The drawing under review shows one solid part. Ordinate dimensions are in mm from its lowest x, y, z. A direction names the side the tool comes from. Round coordinates to 2 decimals unless told otherwise and drop trailing zeros. Write each loop counter-clockwise with the first axis right and the second up, starting at its lowest first coordinate (ties: lowest second). Pieces come first, ordered by that corner, then holes. Notation, with made-up numbers: (-22.75, -29) -> (12.25, -29) arc R13 ccw to (12.25, -9) -> close; hole circle Ø4 at (83, 34.25). An arc over 180 degrees is marked (long way). Answer in a Markdown table with one row per item.
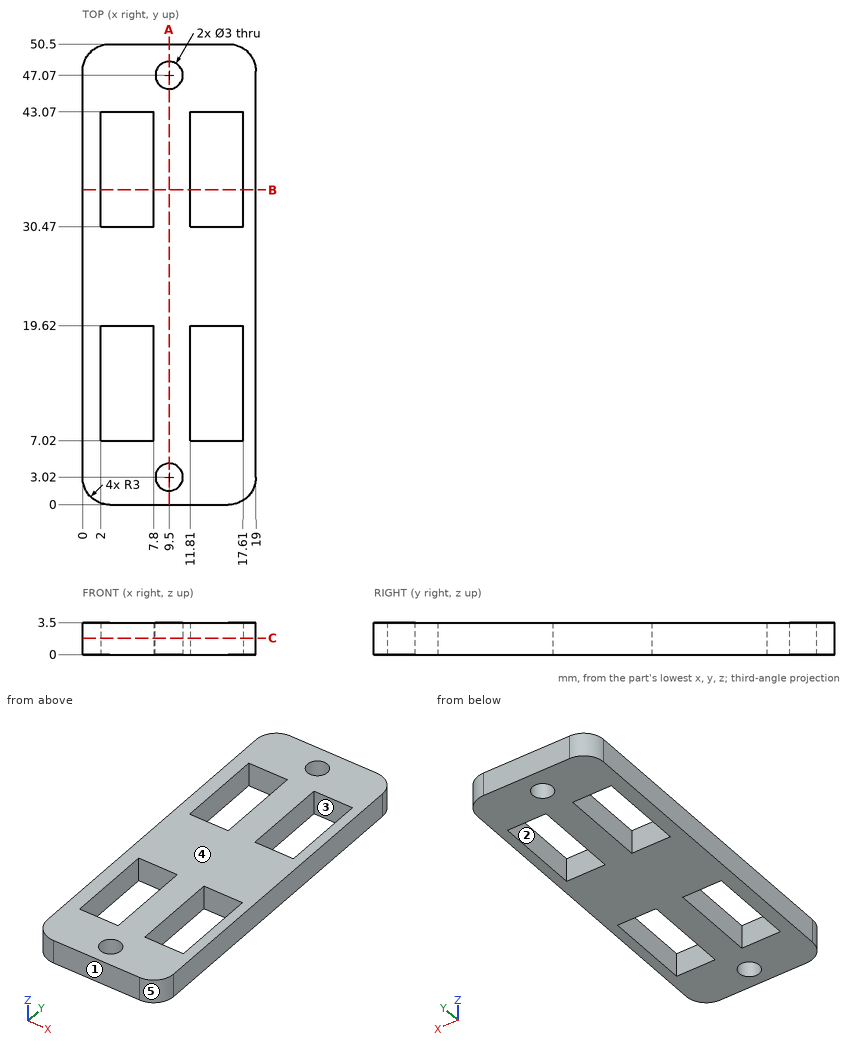
1) Consider section B-B on y = 34.5. State the section outline as (x, z) points.
Solved:
| item | result |
|---|---|
| outline | (0, 0) -> (2, 0) -> (2, 3.5) -> (0, 3.5) -> close; (7.8, 0) -> (11.81, 0) -> (11.81, 3.5) -> (7.8, 3.5) -> close; (17.61, 0) -> (19, 0) -> (19, 3.5) -> (17.61, 3.5) -> close |
2) For the marked faces 1 and 2, list the 3-axis set-ups (+Z, -Z, +X, -X, +Y, -Y) from which the entire face can be reached by the end or side of a thin tool; tool diameter is ignored.
Solved:
| item | result |
|---|---|
| face 1 | +Z, -Z, +X, -X, -Y |
| face 2 | +Z, -Z |
3) Consider section C-C on z = 1.8. State the section outline as (x, y) points, then the cut area to 3 significant figures.
Solved:
| item | result |
|---|---|
| outline | (0, 3) arc R3 ccw to (3, 0) -> (16, 0) arc R3 ccw to (19, 3) -> (19, 47.5) arc R3 ccw to (16, 50.5) -> (3, 50.5) arc R3 ccw to (0, 47.5) -> close; hole (2, 7.02) -> (7.8, 7.02) -> (7.8, 19.62) -> (2, 19.62) -> close; hole (2, 30.47) -> (7.8, 30.47) -> (7.8, 43.07) -> (2, 43.07) -> close; hole circle Ø3 at (9.5, 3.02); hole circle Ø3 at (9.5, 47.07); hole (11.81, 7.02) -> (17.61, 7.02) -> (17.61, 19.62) -> (11.81, 19.62) -> close; hole (11.81, 30.47) -> (17.61, 30.47) -> (17.61, 43.07) -> (11.81, 43.07) -> close |
| area | 645 mm² |
4) For line 1 (X direction, y = 34.5, z = 1.35); line 2 (Y direction, x = 14.5, z = 1.95); line 3 (Y direction, x = 9.5, z = 2.05), list the stretches that pass through material, from the lowest coordinate up. Write a range as [from, to].
Solved:
| item | result |
|---|---|
| line 1 | [0, 2], [7.8, 11.81], [17.61, 19] |
| line 2 | [0, 7.02], [19.62, 30.47], [43.07, 50.5] |
| line 3 | [0, 1.52], [4.52, 45.57], [48.57, 50.5] |
5) Mouldability with a two-part tool opening along Y and no side actions: class the marked faces 3, 4 and 5 as pulls with the +Y half, pulls with the -Y half, needs draft (parallel to the pull), parting line crosses it, or undercut.
Solved:
| item | result |
|---|---|
| face 3 | undercut |
| face 4 | needs draft |
| face 5 | pulls with the -Y half |
6) Consider section A-A on x = 9.5. State the section outline as (y, z) points.
Solved:
| item | result |
|---|---|
| outline | (0, 0) -> (1.52, 0) -> (1.52, 3.5) -> (0, 3.5) -> close; (4.52, 0) -> (45.57, 0) -> (45.57, 3.5) -> (4.52, 3.5) -> close; (48.57, 0) -> (50.5, 0) -> (50.5, 3.5) -> (48.57, 3.5) -> close |
